Work out the finished part from the listing and answer in its coordinate system (mm). Face numbers are marked on the shaded views. A direction names the side the tool comes from. Give positions to 0.01 mm unless a question says otherwise; leave off trailing zeros. Order: outer loops, then holes, each group sorted by start corner. A loop starts at its lowest first (then second) coordinate and runs counter-clockwise, first axis right, second up.
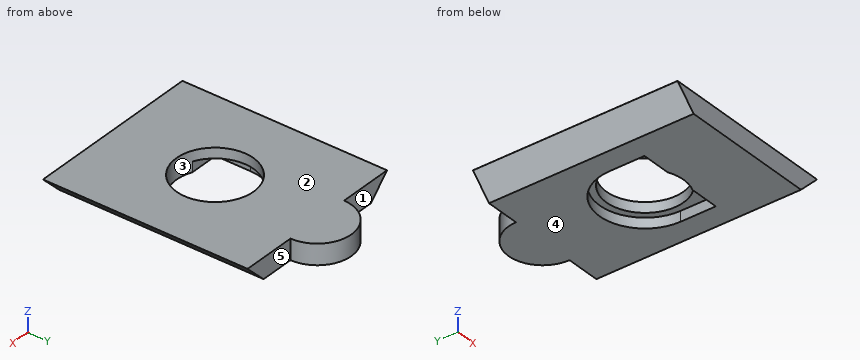
```python
from build123d import *

# Parameters (mm, degrees)
PAD028_DEPTH            = 3
POCKET013_DEPTH         = 1.5
CHAMFER_SIZE            = 2.99
SKETCH061_R             = 5.65
POCKET017_DEPTH         = 3.001
BODY019_PLACEMENT_ANGLE = 180


with BuildPart() as part:
    # Sketch057 → Pad028 (new body)
    with BuildSketch(Plane.XY):
        with BuildLine():
            Line((-13, 15), (-5, 15))
            ThreePointArc((5, 15), (0, 20), (-5, 15))
            Line((5, 15), (13, 15))
            Line((13, 15), (13, -15))
            Line((13, -15), (-13, -15))
            Line((-13, -15), (-13, 15))
        make_face()
    extrude(amount=-PAD028_DEPTH)

    # Sketch056 → Pocket013 (cut)
    with BuildSketch(Plane.XY):
        with BuildLine():
            ThreePointArc((6.65, 0), (0, 6.65), (-6.65, 0))
            Line((-6.65, -5.15), (-6.65, 0))
            Line((6.65, -5.15), (-6.65, -5.15))
            Line((6.65, 0), (6.65, -5.15))
        make_face()
    extrude(amount=-POCKET013_DEPTH, mode=Mode.SUBTRACT)

    # Chamfer
    chamfer_edges = [part.edges().sort_by_distance(p)[0] for p in [
        (-13, 0, 0),
        (13, 0, 0),
    ]]
    chamfer(chamfer_edges, length=CHAMFER_SIZE)

    # Sketch061 → Pocket017 (cut, through all)
    with BuildSketch(Plane.XY):
        Circle(SKETCH061_R)
    extrude(amount=-POCKET017_DEPTH, mode=Mode.SUBTRACT)


with BuildPart() as part_1:
    # Body019 placement: moved
    add(part.part.moved(Location((0, 0, 0.4))).rotate(Axis((0, 0, 0.4), (0, 1, 0)), BODY019_PLACEMENT_ANGLE))


solid = part_1.part
```
1. Which of the six approach directions +Z, -Z, +X, -X, +Y, -Y give full straight-line access (tool end or side, diameter ignored) to the marked faces 1 and 2?
Findings below:
face 1: +Z, -Z, -X, +Y
face 2: +Z, +X, -X, +Y, -Y
2. The part is cut by section A-A (x = 0). Write down the section's boundary in (y, z).
Findings below:
outline: (-15, 0.4) - (-5.65, 0.4) - (-5.65, 3.4) - (-15, 3.4) - close; (5.65, 1.9) - (6.65, 1.9) - (6.65, 0.4) - (20, 0.4) - (20, 3.4) - (5.65, 3.4) - close
3. The part is cut by section B-B (z = 0.8). Write down the section's boundary in (x, y), then the cut area to 3 significant figures.
Findings below:
outline: (-10.41, -15) - (10.41, -15) - (10.41, 15) - (5, 15) arc R5 ccw to (-5, 15) - (-10.41, 15) - close; hole (-6.65, -5.15) - (-2.32, -5.15) arc R5.65 ccw to (2.32, -5.15) - (6.65, -5.15) - (6.65, 0) arc R6.65 ccw to (-6.65, 0) - close
area: 524 mm2
4. The mould has two halves that part along Y. Classify the marked faces 3, 4 and 5: pulls with the +Y half, pulls with the -Y half, needs draft (parallel to the pull), parting line crosses it, or undercut.
Findings below:
face 3: undercut
face 4: needs draft
face 5: pulls with the +Y half
5. Given P1, Ø1.5, axis at x = -8.5, z = 1, coming from the +Y side; P2, Ø1.2, axis at x = 3.5, z = 1.5, coming from the +Y side; P3, Ø1.6, axis at y = -2.5, z = 1, coming from the -X side, each flat-ended and moving along its own axis, determine where each tip first touches the part or whether it passes through.
Findings below:
P1: stops at y = 15
P2: stops at y = 19.07
P3: stops at x = -11.41
6. Straight lines are drawn through the part: probe 1 along Y at (x, z) = (0, 2.55); probe 2 along Y at (x, z) = (0, 1.7); probe 3 along X at (y, z) = (0, 2). For each, find the intervals that lie inside material, in ascending order.
Findings below:
probe 1: y = -15 to -5.65, 5.65 to 20
probe 2: y = -15 to -5.65, 6.65 to 20
probe 3: x = -11.61 to -5.65, 5.65 to 11.61
